Can you work these out from the model? Positions are in its coordinate system, mm. A direction names the side the tool comes from. Coordinates: 2 decimals unless noted, no trailing zeros. Order: outer loops, then holes, each group sorted by start corner. A loop starts at its lowest first (then second) coordinate and runs counter-clockwise, first axis right, second up. Notation, with made-up numbers: (15.25, 85.25) - (44.25, 85.25) arc R17 ccw to (44.25, 100.25) - close; hole circle Ø3 at (-20.5, 0). An arc over 180 degrees is marked (long way). Use a Markdown table: item, result. Add a question column.
(1) I want a section at B-B (z = 0). List the corners of the cut face in (x, y) for me, and give its area (3 significant figures).
(2) On a 3-axis mill with a long thin cutter (end or side, diameter ignored), from which of +Z, -Z, +X, -X, +Y, -Y can I reach the whole of each face in a straight line? I mean faces 1 (the flat face through (10, 89, -6)), 2 (the flat face through (-4.15, 89, 7)). Say none if no direction works.
(3) If I drill on L1, parallel to Z at x = 9.25, y = 164; L2, parallel to Z at x = 0, y = 141.5; L3, parallel to X at y = 17, z = -8.25, over which ranges is the centre line in solid material (lowest first)? Write a range as [from, to].
(4) I want a section at A-A (x = 7). List the corners of the cut face in (y, z) for me.
(5) We'd pull the mould along X, two halves only. Please class faces 3 (the flat face through (4.15, 89, -7)), 4 (the flat face through (10, 89, 6)), 5 (the flat face through (-10, 89, -6)), 6 (the flat face through (-2, 180, 0)): pulls with the +X half, pulls with the -X half, needs draft (parallel to the pull), parting line crosses it, or undercut.
Autodesk Inventor part; units mm, degrees
ref_plane "YZ Plane" through (0, 0, 0) normal (1, 0, 0) x (0, 1, 0)
ref_plane "XZ Plane" through (0, 0, 0) normal (0, 1, 0) x (-1, 0, 0)
ref_plane "XY Plane" through (0, 0, 0) normal (0, 0, 1) x (1, 0, 0)
sketch "草圖1" plane through (0, 0, 0) normal (0, 1, 0) x (-1, 0, 0)
  line L0 (10, 10) -> (10, -10)
  line L1 (-10, -10) -> (-10, 10)
  line L2 (-10, 10) -> (10, -10) construction
  line L3 (10, 10) -> (-10, -10) construction
  line L4 (2.65, -10) -> (2.65, -8.5)
  line L5 (2.65, -8.5) -> (4.15, -8.5)
  line L6 (4.15, -8.5) -> (4.15, -4.9973)
  arc A0 (4.15, -4.9973) -> (-4.15, -4.9973) centre (0, -10) ccw
  line L7 (0, -10) -> (0, 0) construction
  line L8 (-2.65, -10) -> (-2.65, -8.5)
  line L9 (-2.65, -8.5) -> (-4.15, -8.5)
  line L10 (-4.15, -8.5) -> (-4.15, -4.9973)
  arc A1 (4.9973, 4.15) -> (4.9973, -4.15) centre (10, 0) ccw
  line L11 (10, 2.65) -> (8.5, 2.65)
  line L12 (8.5, 2.65) -> (8.5, 4.15)
  line L13 (8.5, 4.15) -> (4.9973, 4.15)
  line L14 (10, -2.65) -> (8.5, -2.65)
  line L15 (8.5, -2.65) -> (8.5, -4.15)
  line L16 (8.5, -4.15) -> (4.9973, -4.15)
  arc A2 (-4.15, 4.9973) -> (4.15, 4.9973) centre (0, 10) ccw
  line L17 (-2.65, 10) -> (-2.65, 8.5)
  line L18 (-2.65, 8.5) -> (-4.15, 8.5)
  line L19 (-4.15, 8.5) -> (-4.15, 4.9973)
  line L20 (2.65, 10) -> (2.65, 8.5)
  line L21 (2.65, 8.5) -> (4.15, 8.5)
  line L22 (4.15, 8.5) -> (4.15, 4.9973)
  arc A3 (-4.9973, -4.15) -> (-4.9973, 4.15) centre (-10, 0) ccw
  line L23 (-10, -2.65) -> (-8.5, -2.65)
  line L24 (-8.5, -2.65) -> (-8.5, -4.15)
  line L25 (-8.5, -4.15) -> (-4.9973, -4.15)
  line L26 (-10, 2.65) -> (-8.5, 2.65)
  line L27 (-8.5, 2.65) -> (-8.5, 4.15)
  line L28 (-8.5, 4.15) -> (-4.9973, 4.15)
  line L29 (10, -10) -> (2.65, -10)
  line L30 (-2.65, -10) -> (-10, -10)
  line L31 (-10, 10) -> (-2.65, 10)
  line L32 (2.65, 10) -> (10, 10)
  circle A4 centre (0, 0) radius 1.65
  point P0 (2.65, -9.25)
  point P1 (-2.65, -9.25)
  point P2 (9.25, 2.65)
  point P3 (9.25, -2.65)
  point P4 (-2.65, 9.25)
  point P5 (2.65, 9.25)
  point P6 (-9.25, -2.65)
  point P7 (-9.25, 2.65)
  dimension "d0" = 20
  dimension "d1" = 20
  dimension "d2" = 13
  dimension "d3" = 1.5
  dimension "d4" = 2.65
  dimension "d5" = 4.15
  dimension "d8" = 360
  dimension "d10" = 3.3
extrude "擠出1" add sketch "草圖1" along normal blind 180 contours L0 L11 L12 L13 A1 L16 L15 L14 L29 L4 L5 L6 A0 L10 L9 L8 L30 L1 L23 L24 L25 A3 L28 L27 L26 L31 L17 L18 L19 A2 L22 L21 L20 L32
properties part number "j2j3 alumi ext"
Answers follow:
| question | item | result |
|---|---|---|
| 1 | outline | (-3.5, 0) - (-1.65, 0) - (-1.65, 180) - (-3.5, 180) - close; (1.65, 0) - (3.5, 0) - (3.5, 180) - (1.65, 180) - close |
| 1 | area | 666 mm² |
| 2 | face 1 | +Z, -Z, +X, +Y, -Y |
| 2 | face 2 | +Y, -Y |
| 3 | L1 | z = [-10, -2.65], [2.65, 10] |
| 3 | L2 | z = [-3.5, -1.65], [1.65, 3.5] |
| 3 | L3 | x = [-10, -4.15], [4.15, 10] |
| 4 | outline | (0, -10) - (180, -10) - (180, -4.15) - (0, -4.15) - close; (0, 4.15) - (180, 4.15) - (180, 10) - (0, 10) - close |
| 5 | face 3 | undercut |
| 5 | face 4 | pulls with the +X half |
| 5 | face 5 | pulls with the -X half |
| 5 | face 6 | needs draft |
